The listing builds one solid part. Answer for the finished solid, in the listing's coordinates (mm). A direction names the side the tool comes from. Give positions to 0.01 mm unless a question says otherwise; leave off trailing zeros. Loops run counter-clockwise (first coordinate to the right, second up) from the corner with the lowest first, then second, coordinate; pieces in that order, holes last. Notation, with made-up numbers: (-26, -33) - (-10, -33) arc R27 cw to (-10, -9) - close; hole circle Ø1 at (42.25, 54.5). An arc over 180 degrees is marked (long way). Answer in a Markdown table with one row per item. Add a question column.
```python
from build123d import *

# Parameters (mm, degrees)
F0_W     = 2
F0_H     = 5
F0_W_2   = 18
F0_H_2   = 2
F1_DEPTH = 6
F2_R     = 0.99999
F3_R     = 1
F4_R     = 0.99999


# Not quite as in the source:
# - a fillet or chamfer is up to 0.001 mm smaller than in the source, because OpenCascade refuses the exact size


with BuildPart() as f1:
    # F0 (on Top) → F1 (new body)
    with BuildSketch(Plane.XY):
        with Locations((1, 2.5)):
            Rectangle(F0_W, F0_H)
        with Locations((11, -1)):
            Rectangle(F0_W_2, F0_H_2)
        Polygon((2, 0), (0, 0), (0, -11), (2, -11), (2, -2), align=None)
    extrude(amount=F1_DEPTH)

    # F2 (radius 1 in the source; OpenCascade refuses exactly that, so slightly less here)
    f2_edges = [f1.edges().sort_by_distance(p)[0] for p in [
        (0, 5, 3),
        (2, 5, 3),
    ]]
    fillet(f2_edges, radius=F2_R)

    # F3
    f3_edges = [f1.edges().sort_by_distance(p)[0] for p in [
        (0, -11, 3),
    ]]
    fillet(f3_edges, radius=F3_R)

    # F4 (radius 1 in the source; OpenCascade refuses exactly that, so slightly less here)
    f4_edges = [f1.edges().sort_by_distance(p)[0] for p in [
        (2, -11, 3),
    ]]
    fillet(f4_edges, radius=F4_R)


solid = f1.part
```
(1) The mould has two halves that part along X. Classify faces 1 (the face through (1.699, -10.715, 3.042)), 2 (the face through (5.5, -1.8, 0)), 3 (the face through (0.285, -10.699, 3.042)): pulls with the +X half, pulls with the -X half, needs draft (parallel to the pull), parting line crosses it, or undercut.
(2) A cutting plane is placed at C-C on y = -7.25. Determine the outline of the cut face in (x, z), plus the area to 3 significant figures.
(3) A tool of negligible diameter and unlimited length cuts with its end or side. For faces 4 (the face through (2, 2, 3)), 5 (the face through (0, -3, 3)), 6 (the face through (2, -6, 3)), from which of +Z, -Z, +X, -X, +Y, -Y can it reach the whole face along a straight path? Write none if from no direction.
(4) Find the intervals of material crossed by line 1 along X through (y, z) = (2, 1.65); line 2 along Y through (x, z) = (3, 0.65), in increasing order. Write a range as [from, to].
(5) Given pin 1 Ø2 at (x, z) = (8, 2.5) entering from +Y; pin 2 Ø1.2 at (y, z) = (1.5, 2) entering from +X, each flat-ended and moving along its own axis, determine where each tip first touches the part or whether it passes through.
(6) A cutting plane is placed at B-B on x = 11.5. Determine the outline of the cut face in (y, z).
Evaluation:
| question | item | result |
|---|---|---|
| 1 | face 1 | pulls with the +X half |
| 1 | face 2 | needs draft |
| 1 | face 3 | pulls with the -X half |
| 2 | outline | (0, 0) - (2, 0) - (2, 6) - (0, 6) - close |
| 2 | area | 12.0 mm² |
| 3 | face 4 | +Z, -Z, +X, +Y |
| 3 | face 5 | +Z, -Z, -X, +Y, -Y |
| 3 | face 6 | +Z, -Z, +X, -Y |
| 4 | line 1 | x = [0, 2] |
| 4 | line 2 | y = [-2, 0] |
| 5 | pin 1 | stops at y = 0 |
| 5 | pin 2 | stops at x = 2 |
| 6 | outline | (-2, 0) - (0, 0) - (0, 6) - (-2, 6) - close |
